from build123d import *

# Parameters (mm, degrees)
F0_R     = 31.75
F1_DEPTH = 106.68
F4_R     = 39.37
F5_DEPTH = 12.7
F6_R     = 4.953
F7_DEPTH = 25.654


with BuildPart() as f1:
    # F0 (on Top) → F1 (new body)
    with BuildSketch(Plane.XY):
        Circle(F0_R)
    extrude(amount=F1_DEPTH)

    # F4 (on face) → F5 (join)
    with BuildSketch(Plane(origin=(0, 0, 0), x_dir=(0, -1, 0), z_dir=(-1, 0, 0))):
        with Locations((0, 142.158583)):
            Circle(F4_R)
    extrude(amount=F5_DEPTH)

    # F6 (on face) → F7 (join)
    with BuildSketch(Plane(origin=(-12.7, 0, 0), x_dir=(0, -1, 0), z_dir=(-1, 0, 0))):
        with Locations((0, 142.158583)):
            Circle(F6_R)
    extrude(amount=F7_DEPTH)


solid = f1.part
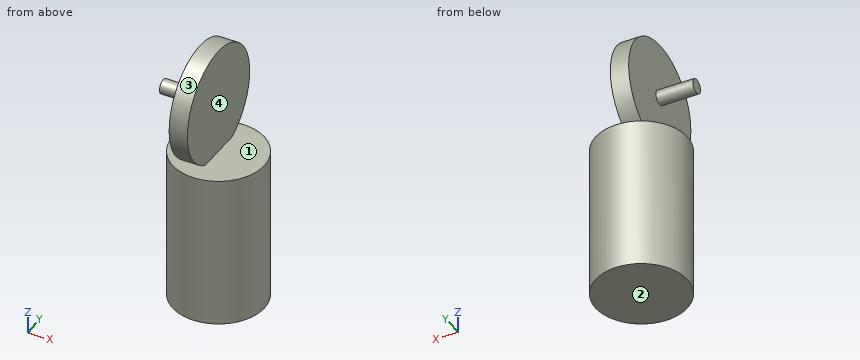
Geometry: final body of the model. Coordinates: model frame, mm. Face numbers are marked on the shaded views. Give positions to 0.01 mm unless a question says otherwise; leave off trailing zeros. Loops run counter-clockwise (first coordinate to the right, second up) from the corner with the lowest first, then second, coordinate; pieces in that order, holes last. Notation, with made-up numbers: (32.5, 56.25) - (43.5, 56.25) arc R24 ccw to (43.5, 94.25) - close; hole circle Ø3 at (65.25, -26.5). An arc over 180 degrees is marked (long way). Answer as CSV lines item,"result". Start each with the question number.
1. Pin query (flat end, axial travel): P1, Ø5, axis at y = 18, z = 35, coming from the +X side; P2, Ø1, axis at y = 13.5, z = 116.5, coming from the +X side; P3, Ø10, axis at x = 17.5, z = 65, coming from the -Y side. Return the tip coordinate at first contact, or that it passes through.
2. Section D-D, the plane x = 14. Return loops of the section in (y, z), plus the area to 3 significant figures.
3. Section A-A, the plane y = 27.5. Return loops of the section in (x, z).
4. Section B-B, the plane z = 139. Return loops of the section in (x, y), plus the area to 3 significant figures.
5. Draft query along Z for the marked faces 1, 2, 3 and 4. Return one class per face: released by +Z, released by -Z, zero draft, split by the parting line, or undercut.
6. Ray query, L1, parallel to X at y = 0.5, z = 45; L2, parallel to X at y = -28, z = 169; L3, parallel to Z at x = 23, y = -10. Return the intervals inside material, ascending.
7. Section C-C, the plane y = 0. Return loops of the section in (x, z), plus the area to 3 significant figures.
Answers:
1,P1,"stops at x = 27.71"
1,P2,"stops at x = 0"
1,P3,"stops at y = -29.19"
2,outline,"(-28.5, 0) - (28.5, 0) - (28.5, 106.68) - (-28.5, 106.68) - close"
2,area,"6,080 mm2"
3,outline,"(-15.87, 0) - (15.87, 0) - (15.87, 106.68) - (-15.87, 106.68) - close; (-12.7, 113.99) - (0, 113.99) - (0, 170.33) - (-12.7, 170.33) - close"
4,outline,"(-38.35, -3.82) - (-12.7, -3.82) - (-12.7, -39.24) - (0, -39.24) - (0, 39.24) - (-12.7, 39.24) - (-12.7, 3.82) - (-38.35, 3.82) - close"
4,area,"1,190 mm2"
5,face 1,"undercut"
5,face 2,"released by -Z"
5,face 3,"undercut"
5,face 4,"zero draft"
6,L1,"x = -31.75 to 31.75"
6,L2,"x = -12.7 to 0"
6,L3,"z = 0 to 106.68"
7,outline,"(-38.35, 137.21) - (-12.7, 137.21) - (-12.7, 106.68) - (-31.75, 106.68) - (-31.75, 0) - (31.75, 0) - (31.75, 106.68) - (0, 106.68) - (0, 181.53) - (-12.7, 181.53) - (-12.7, 147.11) - (-38.35, 147.11) - close"
7,area,"7,980 mm2"
